Could you check a few things on this model? Use its own coordinates, in mm. Face numbers are marked on the shaded views. A direction names the side the tool comes from. Round coordinates to 2 decimals unless told otherwise and drop trailing zeros. Loops run counter-clockwise (first coordinate to the right, second up) from the corner with the lowest first, then second, coordinate; pieces in that order, holes last. Notation, with made-up numbers: (72.5, 11.5) -> (103.5, 11.5) arc R7 cw to (103.5, 19.5) -> close; hole circle Ø11 at (51, 87.25). An arc over 180 degrees is marked (long way). One line per item, written item: value.
from build123d import *

# Parameters (mm, degrees)
SKETCH7_W           = 30
SKETCH7_H           = 30
SKETCH7_W_2         = 25
SKETCH7_H_2         = 25
SKETCH8_R           = 20
BOSS_EXTRUDE1_DEPTH = 30
SKETCH9_R           = 10
CUT_EXTRUDE1_DEPTH  = 30
SKETCH13_R          = 3
BOSS_EXTRUDE2_DEPTH = 6


with BuildPart() as part:
    # Sweep4: sweep along a path in Sketch2
    with BuildLine(Plane(origin=(0, 0, 0), x_dir=(0, 0, -1), z_dir=(1, 0, 0))) as sweep4_path:
        Line((-130.5, 0), (0, 0))
        Line((0, 0), (130.5, -226.032630388))
    # Sketch7 → Sweep4 (sweep)
    with BuildSketch(Plane.XY.offset(130.5)):
        Rectangle(SKETCH7_W, SKETCH7_H)
        Rectangle(SKETCH7_W_2, SKETCH7_H_2, mode=Mode.SUBTRACT)
    sweep(path=sweep4_path.line, transition=Transition.RIGHT)

    # Sketch8 → Boss-Extrude1 (add)
    with BuildSketch(Plane(origin=(15, 0, 0), x_dir=(0, 0, -1), z_dir=(1, 0, 0))):
        Circle(SKETCH8_R)
        with Locations((-130.5, 0)):
            Circle(SKETCH8_R)
        with Locations((130.5, -226.032630388)):
            Circle(SKETCH8_R)
    extrude(amount=-BOSS_EXTRUDE1_DEPTH)

    # Sketch9 → Cut-Extrude1 (cut)
    with BuildSketch(Plane(origin=(15, 0, 0), x_dir=(0, 0, -1), z_dir=(1, 0, 0))):
        with Locations(Location((0, 0, 0), (0, 0, 90))):
            Circle(SKETCH9_R)
        with Locations(Location((-130.5, 0, 0), (0, 0, 90))):
            Circle(SKETCH9_R)
        with Locations(Location((130.5, -226.032630388, 0), (0, 0, 90))):
            Circle(SKETCH9_R)
    extrude(amount=-CUT_EXTRUDE1_DEPTH, mode=Mode.SUBTRACT)

    # Sketch13 → Boss-Extrude2 (add, symmetric)
    with BuildSketch(Plane(origin=(0, 0, 0), x_dir=(0, 0, -1), z_dir=(1, 0, 0))):
        with BuildLine():
            Line((19.604759334, -3.956439237), (9.859578521, 1.669943529))
            ThreePointArc((9.859578521, 1.669943529), (5, 8.660254038), (-3.483575742, 9.373617234))
            Line((-3.483575742, 9.373617234), (-13.228756555, 15))
            ThreePointArc((-13.228756555, 15), (-8.58962126, 18.061517284), (-3.287056594, 19.728032313))
            Line((-3.287056594, 19.728032313), (22.000269373, 63.526965676))
            ThreePointArc((22.000269373, 63.526965676), (29.427887497, 69.154976368), (38.643459087, 67.770326373))
            Line((38.643459087, 67.770326373), (40.285678743, 66.768182028))
            ThreePointArc((40.285678743, 66.768182028), (45.677401844, 59.431654602), (44.366919196, 50.421774031))
            Line((44.366919196, 50.421774031), (18.728505447, 7.017341642))
            ThreePointArc((18.728505447, 7.017341642), (19.936543429, 1.591928422), (19.604759334, -3.956439237))
        make_face()
        with Locations((35, 60.621778265)):
            Circle(SKETCH13_R, mode=Mode.SUBTRACT)
    extrude(amount=BOSS_EXTRUDE2_DEPTH, both=True)


solid = part.part
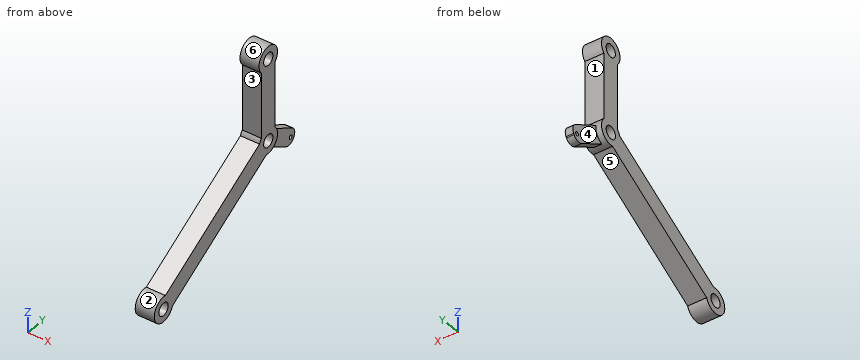
(1) If we section it at B-B, the plane y = 0: Please give me the cut outline in (x, z), then the cut area to 3 significant figures.
Recorded:
outline: (-15, -20) -> (15, -20) -> (15, -10) -> (-15, -10) -> close; (-15, 10) -> (15, 10) -> (15, 120.5) -> (-15, 120.5) -> close; (-15, 140.5) -> (15, 140.5) -> (15, 150.5) -> (-15, 150.5) -> close; hole (-12.5, 20) -> (12.5, 20) -> (12.5, 110.5) -> (-12.5, 110.5) -> close
area: 1,650 mm²
(2) If we section it at C-C, the plane z = 50.5: Please give me the cut outline in (x, y).
Recorded:
outline: (-15, -15) -> (15, -15) -> (15, 15) -> (-15, 15) -> close; hole (-12.5, -12.5) -> (12.5, -12.5) -> (12.5, 12.5) -> (-12.5, 12.5) -> close
(3) For the marked faces 1 and 2, which set-ups out of +Z, -Z, +X, -X, +Y, -Y let a thin tool reach every point of the face, with its end or its side?
Recorded:
face 1: +X, -X, +Y
face 2: +X, -X
(4) If we section it at A-A, the plane z = 130.5: Please give me the cut outline in (x, y).
Recorded:
outline: (-15, -20) -> (15, -20) -> (15, -10) -> (-15, -10) -> close; (-15, 10) -> (15, 10) -> (15, 20) -> (-15, 20) -> close
(5) I'm going to push flat-ended pins straight in: pin 1 Ø1.5 at (x, y) = (-4.5, -104) entering from +Z; pin 2 Ø12 at (x, z) = (0, 111) entering from +Y; pin 3 Ø3 at (x, z) = (5.5, 4.5) entering from +Y; pin 4 Ø16 at (y, z) = (0, 130.5) entering from -X. Where does each tip first touch, or does it pass through?
Recorded:
pin 1: z = -42.29
pin 2: y = 15
pin 3: y = 20.23
pin 4: through
(6) Thinking about a two-plate mould opening in Z: for the marked faces 3, 4, 5 and 6, which applies, released by +Z, released by -Z, zero draft, split by the parting line, or undercut?
Recorded:
face 3: undercut
face 4: zero draft
face 5: released by -Z
face 6: undercut
(7) If I drill on L1, parallel to Z at x = 1.75, y = 0; L2, parallel to Y at x = -7, z = 84.5; L3, parallel to Y at x = 8, z = -125, over which ranges is the centre line in solid material (lowest first)?
Recorded:
L1: -20 to -10, 10 to 20, 110.5 to 120.5, 140.5 to 150.5
L2: -15 to -12.5, 12.5 to 15
L3: -245.26 to -234.38, -217.68 to -206.8, -191.51 to -186.51
(8) If we section it at D-D, the plane y = -101: Please give me the cut outline in (x, z).
Recorded:
outline: (-15, -75.63) -> (15, -75.63) -> (15, -40.99) -> (-15, -40.99) -> close; hole (-12.5, -72.75) -> (12.5, -72.75) -> (12.5, -43.88) -> (-12.5, -43.88) -> close
